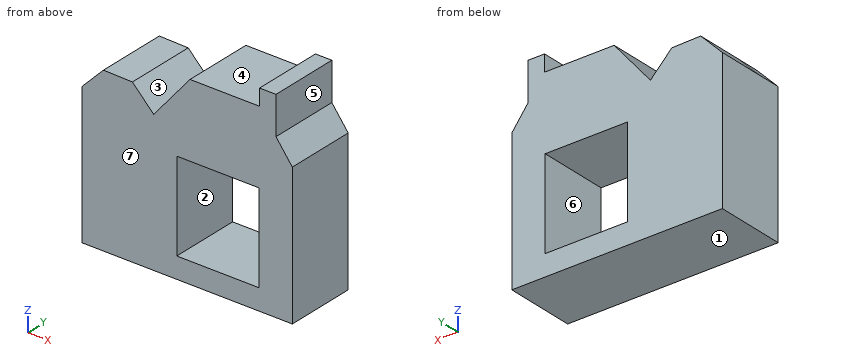
```python
from build123d import *

# Parameters (mm, degrees)
F0_W      = 89.1198969167
F0_H      = 97.0041044056
F0_W_2    = 77.9982568039
F0_H_2    = 151.6424641013
F1_DEPTH  = 25.4
F2_DEPTH  = 25.4
F3_DEPTH  = 25.4
F4_DEPTH  = 25.4
F1_FACE_W = 89.1198969167
F1_FACE_H = 97.0041044056
F3_FACE_W = 89.1198969167
F3_FACE_H = 97.0041044056
F5_DEPTH  = 25.4


with BuildPart() as f1:
    # F0 (on Front) → F1 (new body)
    with BuildSketch(Plane.XZ):
        Polygon((-35.6096097335, 122.5330978632), (-74.9657242284, 74.9862343073), (75.3956741586, 75.7750719786), (57.6258252308, 99.1540849209), (39.8559763029, 122.5330978632), align=None)
        Polygon((75.3956741586, 75.7750719786), (-74.9657242284, 74.9862343073), (-74.9657242284, -76.656229794), (75.3956741586, -76.656229794), align=None)
        with Locations((-5.4095645109, -5.4363291711)):
            Rectangle(F0_W, F0_H, mode=Mode.SUBTRACT)
        with Locations((-113.9648526304, -0.8349977434)):
            Rectangle(F0_W_2, F0_H_2)
        Polygon((-152.9639810324, 74.9862343073), (-74.9657242284, 74.9862343073), (-98.1215983629, 98.4429121017), (-129.5073032379, 99.103666842), align=None)
        Polygon((39.8559763029, 140.2747780085), (39.8559763029, 122.5330978632), (57.6258252308, 99.1540849209), (57.6258252308, 140.2747780085), align=None)
    extrude(amount=F1_DEPTH)

    # F0 (on Front) → F2 (join)
    with BuildSketch(Plane.XZ):
        Polygon((-35.6096097335, 122.5330978632), (-74.9657242284, 74.9862343073), (75.3956741586, 75.7750719786), (57.6258252308, 99.1540849209), (39.8559763029, 122.5330978632), align=None)
        Polygon((75.3956741586, 75.7750719786), (-74.9657242284, 74.9862343073), (-74.9657242284, -76.656229794), (75.3956741586, -76.656229794), align=None)
        with Locations((-5.4095645109, -5.4363291711)):
            Rectangle(F0_W, F0_H, mode=Mode.SUBTRACT)
        with Locations((-113.9648526304, -0.8349977434)):
            Rectangle(F0_W_2, F0_H_2)
        Polygon((-152.9639810324, 74.9862343073), (-74.9657242284, 74.9862343073), (-98.1215983629, 98.4429121017), (-129.5073032379, 99.103666842), align=None)
        Polygon((39.8559763029, 140.2747780085), (39.8559763029, 122.5330978632), (57.6258252308, 99.1540849209), (57.6258252308, 140.2747780085), align=None)
    extrude(amount=F2_DEPTH)

    # F0 (on Front) → F3 (join)
    with BuildSketch(Plane.XZ):
        Polygon((-35.6096097335, 122.5330978632), (-74.9657242284, 74.9862343073), (75.3956741586, 75.7750719786), (57.6258252308, 99.1540849209), (39.8559763029, 122.5330978632), align=None)
        Polygon((75.3956741586, 75.7750719786), (-74.9657242284, 74.9862343073), (-74.9657242284, -76.656229794), (75.3956741586, -76.656229794), align=None)
        with Locations((-5.4095645109, -5.4363291711)):
            Rectangle(F0_W, F0_H, mode=Mode.SUBTRACT)
        with Locations((-113.9648526304, -0.8349977434)):
            Rectangle(F0_W_2, F0_H_2)
        Polygon((-152.9639810324, 74.9862343073), (-74.9657242284, 74.9862343073), (-98.1215983629, 98.4429121017), (-129.5073032379, 99.103666842), align=None)
        Polygon((39.8559763029, 140.2747780085), (39.8559763029, 122.5330978632), (57.6258252308, 99.1540849209), (57.6258252308, 140.2747780085), align=None)
    extrude(amount=-F3_DEPTH)

    # F0 (on Front) → F4 (join)
    with BuildSketch(Plane.XZ):
        Polygon((-35.6096097335, 122.5330978632), (-74.9657242284, 74.9862343073), (75.3956741586, 75.7750719786), (57.6258252308, 99.1540849209), (39.8559763029, 122.5330978632), align=None)
        Polygon((75.3956741586, 75.7750719786), (-74.9657242284, 74.9862343073), (-74.9657242284, -76.656229794), (75.3956741586, -76.656229794), align=None)
        with Locations((-5.4095645109, -5.4363291711)):
            Rectangle(F0_W, F0_H, mode=Mode.SUBTRACT)
        with Locations((-113.9648526304, -0.8349977434)):
            Rectangle(F0_W_2, F0_H_2)
        Polygon((-152.9639810324, 74.9862343073), (-74.9657242284, 74.9862343073), (-98.1215983629, 98.4429121017), (-129.5073032379, 99.103666842), align=None)
        Polygon((39.8559763029, 140.2747780085), (39.8559763029, 122.5330978632), (57.6258252308, 99.1540849209), (57.6258252308, 140.2747780085), align=None)
    extrude(amount=-F4_DEPTH)

    # F0 (on Front) + F1_face (on face) + F3_face (on face) → F5 (join)
    with BuildSketch(Plane.XZ):
        Polygon((39.8559763029, 140.2747780085), (39.8559763029, 122.5330978632), (57.6258252308, 99.1540849209), (57.6258252308, 140.2747780085), align=None)
        Polygon((-152.9639810324, 74.9862343073), (-74.9657242284, 74.9862343073), (-98.1215983629, 98.4429121017), (-129.5073032379, 99.103666842), align=None)
        Polygon((-35.6096097335, 122.5330978632), (-74.9657242284, 74.9862343073), (75.3956741586, 75.7750719786), (57.6258252308, 99.1540849209), (39.8559763029, 122.5330978632), align=None)
        with Locations((-113.9648526304, -0.8349977434)):
            Rectangle(F0_W_2, F0_H_2)
        Polygon((75.3956741586, 75.7750719786), (-74.9657242284, 74.9862343073), (-74.9657242284, -76.656229794), (75.3956741586, -76.656229794), align=None)
        with Locations((-5.4095645109, -5.4363291711)):
            Rectangle(F0_W, F0_H, mode=Mode.SUBTRACT)
    with BuildSketch(Plane(origin=(-42.5421584691, -25.4, 21.4383649256), x_dir=(1, 0, 0), z_dir=(0, -1, 0))):
        Polygon((117.9378326277, 54.336707053), (100.1679836999, 77.7157199953), (100.1679836999, 118.8364130829), (82.398134772, 118.8364130829), (82.398134772, 101.0947329376), (6.9325487356, 101.0947329376), (-32.4235657593, 53.5478693817), (-55.5794398938, 77.0045471761), (-86.9651447688, 77.6653019164), (-110.4218225632, 53.5478693817), (-110.4218225632, -98.0945947196), (117.9378326277, -98.0945947196), align=None)
        with Locations((37.1325939582, -26.8746940967)):
            Rectangle(F1_FACE_W, F1_FACE_H, mode=Mode.SUBTRACT)
    with BuildSketch(Plane(origin=(-42.5421584691, 25.4, 21.4383649256), x_dir=(1, 0, 0), z_dir=(0, 1, 0))):
        Polygon((100.1679836999, -77.7157199953), (117.9378326277, -54.336707053), (117.9378326277, 98.0945947196), (-110.4218225632, 98.0945947196), (-110.4218225632, -53.5478693817), (-86.9651447688, -77.6653019164), (-55.5794398938, -77.0045471761), (-32.4235657593, -53.5478693817), (6.9325487356, -101.0947329376), (82.398134772, -101.0947329376), (82.398134772, -118.8364130829), (100.1679836999, -118.8364130829), align=None)
        with Locations((37.1325939582, 26.8746940967)):
            Rectangle(F3_FACE_W, F3_FACE_H, mode=Mode.SUBTRACT)
    extrude(amount=F5_DEPTH, dir=(0, -1, 0))


solid = f1.part
```
Geometry: final body of the model. Coordinates: model frame, mm. Face numbers are marked on the shaded views. A direction names the side the tool comes from. Round coordinates to 2 decimals unless told otherwise and drop trailing zeros. Loops run counter-clockwise (first coordinate to the right, second up) from the corner with the lowest first, then second, coordinate; pieces in that order, holes last.
Item 1: Line query: L1, parallel to X at y = 19, z = -49; L2, parallel to Z at x = -11, y = -9; L3, parallel to Z at x = -45, y = -10. Output: solid intervals per line, ascending.
Checked values:
L1: x = -152.96 to -49.97, 39.15 to 75.4
L2: z = -76.66 to -53.94, 43.07 to 122.53
L3: z = -76.66 to -53.94, 43.07 to 111.19
Item 2: Reachability of the marked faces 4, 5, 6 and 7 from +Z, -Z, +X, -X, +Y, -Y: full face, straight path, thin tool, end or side. Return the list, or none.
Checked values:
face 4: +Z, -X, +Y, -Y
face 5: +Z, +X, +Y, -Y
face 6: +Y, -Y
face 7: +Z, -Z, +X, -X, -Y
Item 3: Contact query for flat-ended pins moving along their axis: P1, Ø14, axis at y = -8, z = 130.5, coming from the -X side; P2, Ø1.5, axis at x = -79, y = -27, coming from the +Z side; P3, Ø12.5, axis at y = 0, z = 129.5, coming from the +X side. Output: stop coordinate, or through.
Checked values:
P1: stops at x = 39.86
P2: stops at z = 79.83
P3: stops at x = 57.63
Item 4: Mould query, pull axis Z, two halves, no side actions, for the marked faces 1, 2 and 3. Classes: released by +Z, released by -Z, zero draft, split by the parting line, or undercut.
Checked values:
face 1: released by -Z
face 2: undercut
face 3: released by +Z
Item 5: Section B-B, the plane z = 10.5. Output: boundary loops of the cut face in (x, y).
Checked values:
outline: (-152.96, -50.8) - (-49.97, -50.8) - (-49.97, 25.4) - (-152.96, 25.4) - close; (39.15, -50.8) - (75.4, -50.8) - (75.4, 25.4) - (39.15, 25.4) - close
Item 6: Section A-A, the plane y = -11.5. Output: boundary loops of the cut face in (x, z), plus the area to 3 significant figures.
Checked values:
outline: (-152.96, -76.66) - (75.4, -76.66) - (75.4, 75.78) - (57.63, 99.15) - (57.63, 140.27) - (39.86, 140.27) - (39.86, 122.53) - (-35.61, 122.53) - (-74.97, 74.99) - (-98.12, 98.44) - (-129.51, 99.1) - (-152.96, 74.99) - close; hole (-49.97, -53.94) - (39.15, -53.94) - (39.15, 43.07) - (-49.97, 43.07) - close
area: 33,200 mm2
Item 7: Section C-C, the plane x = 0. Output: boundary loops of the cut face in (y, z).
Checked values:
outline: (-50.8, -76.66) - (25.4, -76.66) - (25.4, -53.94) - (-50.8, -53.94) - close; (-50.8, 43.07) - (25.4, 43.07) - (25.4, 122.53) - (-50.8, 122.53) - close
Item 8: Section D-D, the plane x = -138. Output: boundary loops of the cut face in (y, z), plus the area to 3 significant figures.
Checked values:
outline: (-50.8, -76.66) - (25.4, -76.66) - (25.4, 90.37) - (-50.8, 90.37) - close
area: 12,700 mm2
